from build123d import *

# Parameters (mm, degrees)
F1_DEPTH = 38.1
F2_R     = 12.7
F3_W     = 381
F3_H     = 6.35
F4_DEPTH = 12.7
F5_W     = 343.8676841179
F5_H     = 6.35
F6_DEPTH = 12.7
F7_R     = 12.7
F8_DEPTH = 2.54


with BuildPart() as f1:
    # F0 (on Top) → F1 (new body)
    with BuildSketch(Plane.XY):
        with BuildLine():
            Line((0, 0), (-70.5706194038, -400.2258708242))
            ThreePointArc((-70.5706194038, -400.2258708242), (0, -406.4), (70.5706194038, -400.2258708242))
            Line((70.5706194038, -400.2258708242), (0, 0))
        make_face()
    extrude(amount=-F1_DEPTH)

    # F2
    f2_edges = [f1.edges().sort_by_distance(p)[0] for p in [
        (0, -406.4, 0),
    ]]
    fillet(f2_edges, radius=F2_R)

    # F3 (on face) → F4 (cut)
    with BuildSketch(Plane(origin=(0, 0, 0), x_dir=(-0.1736481777, 0.984807753, 0), z_dir=(0.984807753, 0.1736481777, 0))):
        with Locations((-190.5, -19.05)):
            Rectangle(F3_W, F3_H)
    extrude(amount=-F4_DEPTH, mode=Mode.SUBTRACT)

    # F5 (on face) → F6 (cut)
    with BuildSketch(Plane(origin=(0, 0, 0), x_dir=(-0.1736481777, -0.984807753, 0), z_dir=(-0.984807753, 0.1736481777, 0))):
        with Locations((209.066157941, -19.05)):
            Rectangle(F5_W, F5_H)
    extrude(amount=-F6_DEPTH, mode=Mode.SUBTRACT)

    # F7 (on face) → F8 (cut)
    with BuildSketch(Plane(origin=(0, 0, -38.1), x_dir=(1, 0, 0), z_dir=(0, 0, -1))):
        with Locations((0, 381)):
            Circle(F7_R)
    extrude(amount=-F8_DEPTH, mode=Mode.SUBTRACT)


solid = f1.part
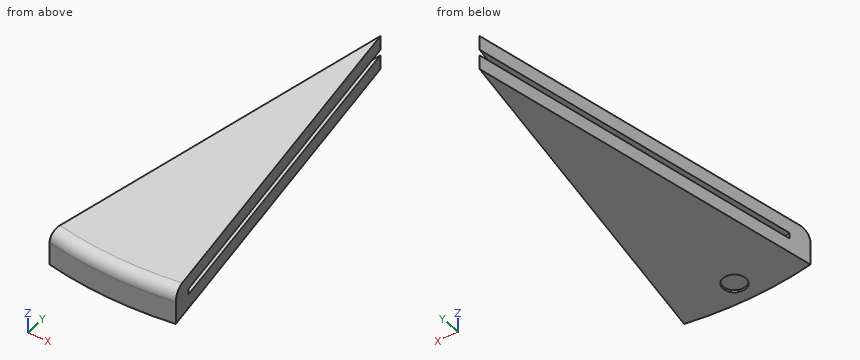
Here's how the part is built. I have some questions about the finished solid (model axes, mm). Give positions to 0.01 mm unless a question says otherwise; leave off trailing zeros. Loops run counter-clockwise (first coordinate to the right, second up) from the corner with the lowest first, then second, coordinate; pieces in that order, holes last. Notation, with made-up numbers: (-11.5, 80) -> (42.5, 80) arc R25 cw to (42.5, 104) -> close; hole circle Ø5 at (1, 48). An arc over 180 degrees is marked (long way). Answer as a JSON object with one key per item and string values. Group by question number.
Item 1: I need wall thicknesses on L1, parallel to Z at x = 24.5, y = -140 (3 decimals); L2, parallel to X at y = -381, z = -36; L3, parallel to X at y = -220, z = -11.5. Which ranges of each line are inside material? Lowest first, please.
Item 2: Imagine slicing it at A-A on y = -381. Write out the boundary of the cut face in (x, z), then the cut area to 3 significant figures.
Item 3: Imagine slicing it at C-C on y = -158.5. Write out the boundary of the cut face in (x, z) (3 decimals).
Item 4: Will these pins go through, and if not, where does the flat tip stop? pin 1 (1 mm diameter, centred on y = -79, z = -15, fed in from -X); pin 2 (4 mm diameter, centred on y = -271.5, z = -26.5, fed in from -X); pin 3 (10 mm diameter, centred on y = -278.5, z = -9.5, fed in from +X).
Item 5: Imagine slicing it at B-B on y = -331.5. Write out the boundary of the cut face in (x, z) (3 decimals), then the cut area to 3 significant figures.
Answer list:
{
 "1": {"L1": "z = -38.1 to -22.225, -15.875 to 0", "L2": "x = -67.18 to -12.7, 12.7 to 67.18", "L3": "x = -38.79 to 38.79"},
 "2": {"outline": "(-67.18, -38.1) -> (-12.7, -38.1) -> (-12.7, -35.56) -> (12.7, -35.56) -> (12.7, -38.1) -> (67.18, -38.1) -> (67.18, 0) -> (-67.18, 0) -> close", "area": "5,050 mm2"},
 "3": {"outline": "(-27.948, -38.1) -> (27.948, -38.1) -> (27.948, -22.225) -> (15.052, -22.225) -> (15.052, -15.875) -> (27.948, -15.875) -> (27.948, 0) -> (-27.948, 0) -> (-27.948, -15.875) -> (-15.052, -15.875) -> (-15.052, -22.225) -> (-27.948, -22.225) -> close"},
 "4": {"pin 1": "stops at x = -14.02", "pin 2": "stops at x = -48.23", "pin 3": "stops at x = 49.99"},
 "5": {"outline": "(-58.452, -38.1) -> (58.452, -38.1) -> (58.452, -22.225) -> (45.556, -22.225) -> (45.556, -15.875) -> (58.452, -15.875) -> (58.452, 0) -> (-58.452, 0) -> (-58.452, -15.875) -> (-45.556, -15.875) -> (-45.556, -22.225) -> (-58.452, -22.225) -> close", "area": "4,290 mm2"}
}
